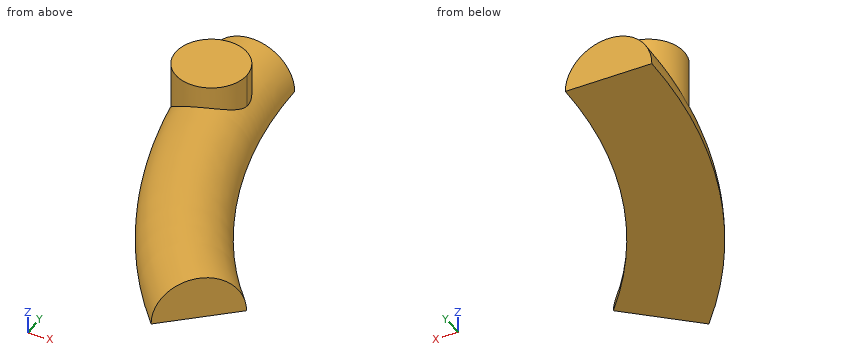
```python
from build123d import *

# Parameters (mm, degrees)
F1_DEPTH = 38.1


with BuildPart() as f1:
    # F0 (on Top) → F1 (new body)
    with BuildSketch(Plane.XY):
        with BuildLine():
            ThreePointArc((0, -22.908895), (-14.689808, -58.373229), (20.774525, -43.683421))
            ThreePointArc((20.774525, -43.683421), (14.689808, -28.993613), (0, -22.908895))
        make_face()
    extrude(amount=F1_DEPTH)

    # F4: sweep along a path in F2
    with BuildLine(Plane.XY) as f4_path:
        ThreePointArc((72.136711, -192.550732), (18.626108, -102.809884), (0, 0))
    # F3 (on Front) → F4 (sweep)
    with BuildSketch(Plane.XZ):
        with BuildLine():
            Line((-25.131127, 0), (25.131127, 0))
            ThreePointArc((25.131127, 0), (0, 25.131127), (-25.131127, 0))
        make_face()
    sweep(path=f4_path.line)


solid = f1.part
```
The listing builds one solid part. Answer for the finished solid, in the listing's coordinates (mm). Give positions to 0.01 mm unless a question says otherwise; leave off trailing zeros. Write each loop counter-clockwise with the first axis right and the second up, starting at its lowest first coordinate (ties: lowest second). Pieces come first, ordered by that corner, then holes. Notation, with made-up numbers: (33, 10.25) -> (91, 10.25) arc R16 ccw to (91, 17.25) -> close; hole circle Ø10 at (-29, -15.5). An arc over 180 degrees is marked (long way). Write item = value, one per line. Start each with the question number.
1) Each of these flat-tipped pins is pushed along its axis until it touches: pin 1 (12 mm diameter, centred on y = -92.5, z = 15, fed in from +X); pin 2 (6 mm diameter, centred on y = -55.5, z = 20.5, fed in from -X); pin 3 (1.5 mm diameter, centred on y = -99.5, z = 10.5, fed in from +X). Where does it stop, or does it pass through?
2) Straight lines are drawn through the part: line 1 along Y through (x, z) = (0.5, 26); line 2 along Y through (x, z) = (-13.5, 24); line 3 along X through (y, z) = (-51.5, 31.5). For each, find the intervals that lie inside material, in ascending order.
3) The part is cut by section A-A, the plane z = 21. Determine the outline of the cut face in (x, y), and give its area (3 significant figures).
Solutions:
q1.pin_1 = 40.65
q1.pin_2 = -18.81
q1.pin_3 = 42.29
q2.line_1 = -64.45 to -22.91
q2.line_2 = -59.47 to -27.89
q2.line_3 = -19.25 to 19.25
q3.outline = (-13.8, 0) arc R306.86 ccw to (-12.6, -27.17) arc R20.77 ccw to (-7.23, -63.16) arc R306.86 ccw to (61.73, -201.62) -> (82.54, -183.48) arc R279.25 cw to (18.79, -52.54) arc R20.77 ccw to (15.39, -29.73) arc R279.25 cw to (13.8, 0) -> close
q3.area = 6,120 mm²
